Can you work these out from the model? Positions are in its coordinate system, mm. Coordinates: 2 decimals unless noted, no trailing zeros. Order: outer loops, then holes, each group sorted by start corner. A loop starts at its lowest first (then second) coordinate and runs counter-clockwise, first axis right, second up. Notation, with made-up numbers: (29.5, 27) - (68.5, 27) arc R25 ccw to (68.5, 55) - close; hole circle Ø5 at (4, -6). An arc over 180 degrees is marked (long way). Return JSON: item names as keys, results as strings. Group by question number.
1) Imagine slicing it at B-B (z = 1.8). Give the number of separate pieces and of enclosed holes in the cut face, and give its area (3 significant figures).
2) Imagine slicing it at A-A (x = -341.5). Write out the boundary of the cut face in (y, z) (3 decimals), and give its area (3 significant figures).
3) If I drill on line 1 along Y through (x, z) = (-67.5, 1.6); line 2 along Y through (x, z) = (-50.8, 2.35); line 3 along X through (y, z) = (-61, 1.3), over which ranges is the centre line in solid material (lowest first)?
4) Imagine slicing it at C-C (y = -105.5). Write out the boundary of the cut face in (x, z) (3 decimals), and give its area (3 significant figures).
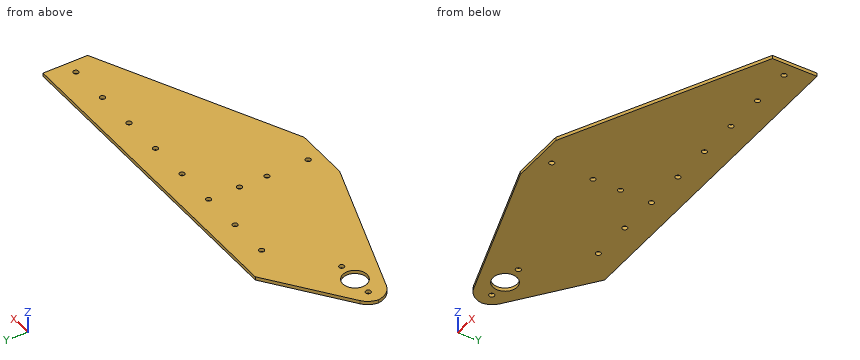
```python
from build123d import *

# Parameters (mm, degrees)
BOSS_EXTRUDE1_DEPTH = 3.175
SKETCH2_R           = 11.176
SKETCH2_R_2         = 2.413
CUT_EXTRUDE1_DEPTH  = 3.175
CHAMFER2_SIZE       = 76.2
CHAMFER2_SIZE2      = 57.420818618
FILLET2_R           = 17.62
SKETCH3_R           = 2.413
CUT_EXTRUDE2_DEPTH  = 3.175


with BuildPart() as part:
    # Sketch1 → Boss-Extrude1 (new body)
    with BuildSketch(Plane.XY):
        Polygon((-304.8, 0), (0, 0), (0, -41.275), (-177.8, -127), (-228.6, -127), (-381, -75.7257486), (-381, 0), align=None)
    extrude(amount=BOSS_EXTRUDE1_DEPTH)

    # Sketch2 → Cut-Extrude1 (cut)
    with BuildSketch(Plane.XY.offset(3.175)):
        with Locations((-349.25, -63.5)):
            Circle(SKETCH2_R)
        with Locations((-279.4, -22.225)):
            Circle(SKETCH2_R_2)
        with Locations((-241.3, -22.225)):
            Circle(SKETCH2_R_2)
        with Locations((-203.2, -22.225)):
            Circle(SKETCH2_R_2)
        with Locations((-203.2, -50.8)):
            Circle(SKETCH2_R_2)
        with Locations((-165.1, -22.225)):
            Circle(SKETCH2_R_2)
        with Locations((-127, -22.225)):
            Circle(SKETCH2_R_2)
        with Locations((-88.9, -22.225)):
            Circle(SKETCH2_R_2)
        with Locations((-12.7, -22.225)):
            Circle(SKETCH2_R_2)
        with Locations((-203.2, -76.2)):
            Circle(SKETCH2_R_2)
        with Locations((-203.2, -114.3)):
            Circle(SKETCH2_R_2)
        with Locations((-50.8, -22.225)):
            Circle(SKETCH2_R_2)
    extrude(amount=-CUT_EXTRUDE1_DEPTH, mode=Mode.SUBTRACT)

    # Chamfer2
    chamfer2_edges = [part.edges().sort_by_distance(p)[0] for p in [
        (-381, 0, 1.5875),
    ]]
    chamfer2_side = [part.faces().sort_by_distance(p)[0] for p in [
        (-190.5, 0, 1.5875),
    ]]
    chamfer(chamfer2_edges, length=CHAMFER2_SIZE, length2=CHAMFER2_SIZE2, reference=chamfer2_side[0])

    # Fillet2
    # the kernel refuses this fillet: 17.62 mm, written as the material it takes off along each edge
    with BuildSketch(Plane(origin=(-381, -75.7257486, -31.65589506), x_dir=(0, 1, 0), z_dir=(0, 0, 1))) as fillet2_piece_1:
        with BuildLine():
            CenterArc((FILLET2_R * 0.718635529169, -FILLET2_R), FILLET2_R, 90, 71.404733131)
            Line((-FILLET2_R * 0.22915922643, -FILLET2_R * 0.681118985733), (0, 0))
            Line((0, 0), (FILLET2_R * 0.718635529169, 0))
        make_face()
    extrude(amount=66.48679012, mode=Mode.SUBTRACT)
    with BuildSketch(Plane(origin=(-381, -57.420818618, -21.962519835), x_dir=(0.7986355100472917, 0.6018150231520498, 0), z_dir=(0, 0, 1))) as fillet2_piece_2:
        with BuildLine():
            CenterArc((FILLET2_R * 0.498581608053, -FILLET2_R), FILLET2_R, 90, 53)
            Line((-FILLET2_R * 0.300053901994, -FILLET2_R * 0.398184976848), (0, 0))
            Line((0, 0), (FILLET2_R * 0.498581608053, 0))
        make_face()
    extrude(amount=47.10003967, mode=Mode.SUBTRACT)

    # Sketch3 → Cut-Extrude2 (cut)
    with BuildSketch(Plane.XY.offset(3.175)):
        with Locations((-368.3, -63.5)):
            Circle(SKETCH3_R)
        with Locations((-330.2, -63.5)):
            Circle(SKETCH3_R)
    extrude(amount=-CUT_EXTRUDE2_DEPTH, mode=Mode.SUBTRACT)


solid = part.part
```
Calculated:
{
 "1": {"separate pieces": "1", "enclosed holes": "14", "area": "34,000 mm2"},
 "2": {"outline": "(-89.015, 0) - (-71.552, 0) - (-71.552, 3.175) - (-89.015, 3.175) - close; (-55.448, 0) - (-27.655, 0) - (-27.655, 3.175) - (-55.448, 3.175) - close", "area": "144 mm2"},
 "3": {"line 1": "-73.82 to 0", "line 2": "-65.77 to -24.64, -19.81 to 0", "line 3": "-380.21 to -360.14, -338.36 to -40.91"},
 "4": {"outline": "(-292.503, 0) - (-133.207, 0) - (-133.207, 3.175) - (-292.503, 3.175) - close", "area": "506 mm2"}
}
